from build123d import *

# Parameters (mm, degrees)
F0_R     = 24
F1_DEPTH = 1000
F2_R     = 20
F3_DEPTH = 1000.001
F4_R     = 10
F5_DEPTH = 25.4


with BuildPart() as f1:
    # F0 (on Front) → F1 (new body)
    with BuildSketch(Plane.XZ):
        Circle(F0_R)
    extrude(amount=-F1_DEPTH)

    # F2 (on Front) → F3 (cut, through all)
    with BuildSketch(Plane.XZ):
        Circle(F2_R)
    extrude(amount=-F3_DEPTH, mode=Mode.SUBTRACT)

    # F4 (on Top) → F5 (cut)
    with BuildSketch(Plane.XY):
        with Locations((0, 100)):
            Circle(F4_R)
    extrude(amount=F5_DEPTH, mode=Mode.SUBTRACT)


solid = f1.part
Work out the finished part from the listing and answer in its coordinate system (mm). A direction names the side the tool comes from. Coordinates: 2 decimals unless noted, no trailing zeros. Write each loop counter-clockwise with the first axis right and the second up, starting at its lowest first coordinate (ties: lowest second). Pieces come first, ordered by that corner, then holes. Notation, with made-up numbers: (66.25, 15.25) - (94.25, 15.25) arc R12 ccw to (94.25, 25.25) - close; hole circle Ø4 at (66, 57.5). An arc over 180 degrees is marked (long way). One line per question, with ' | ' between items.
1) Find section A-A, the plane z = 0. Determine the outline of the cut face in (x, y), and give its area (3 significant figures).
Checks:
outline: (-24, 0) - (-20, 0) - (-20, 1000) - (-24, 1000) - close; (20, 0) - (24, 0) - (24, 1000) - (20, 1000) - close | area: 8,000 mm2
2) Flat-ended cylindrical pins translate along their axes: P1, Ø3, axis at x = 6, y = 146.5, coming from the +Z side; P2, Ø3, axis at x = 12, y = 483.5, coming from the -Z side; P3, Ø10, axis at x = -5, y = 368.5, coming from the -Z side. Find the tip coordinate at first contact, or state that the pin passes through.
Checks:
P1: z = 23.57 | P2: z = -21.58 | P3: z = -24
3) Consider probe 1 along X at (y, z) = (792, -1); probe 2 along Z at (x, y) = (0, 384); probe 3 along X at (y, z) = (66.5, -12.5). Determine where each line is inside the solid, lowest interval first. Write a range as [from, to].
Checks:
probe 1: [-23.98, -19.97], [19.97, 23.98] | probe 2: [-24, -20], [20, 24] | probe 3: [-20.49, -15.61], [15.61, 20.49]
4) Find section D-D, the plane y = 100. Determine the outline of the cut face in (x, z).
Checks:
outline: (-10, 17.32) - (-10, 21.82) arc R24 ccw (long way) to (10, 21.82) - (10, 17.32) arc R20 cw (long way) to start
5) Find section C-C, the plane y = 893. Determine the outline of the cut face in (x, z).
Checks:
outline: circle Ø48 at (0, 0); hole circle Ø40 at (0, 0)
6) The mould has two halves that part along Z. Classify faces 3 (the face through (-5, 1000, 20)), 4 (the face through (-4.336, 493, -19.524)), 5 (the face through (-23.977, 493, 1.055)): +Z half, -Z half, draft (parallel to the pull), parting line (faces both ways), or undercut.
Checks:
face 3: draft | face 4: undercut | face 5: parting line
7) For faces 1 (the face through (-5, 0, 20)), 2 (the face through (-10, 100, 21)), determine the directions among +Z, -Z, +X, -X, +Y, -Y from which every point of the face is accessible in a straight line to the end or side of a thin tool.
Checks:
face 1: +Z, -Z, +X, -X, -Y | face 2: +Z
8) Find section B-B, the plane x = 0. Determine the outline of the cut face in (y, z).
Checks:
outline: (0, -24) - (1000, -24) - (1000, -20) - (0, -20) - close; (0, 20) - (90, 20) - (90, 24) - (0, 24) - close; (110, 20) - (1000, 20) - (1000, 24) - (110, 24) - close
